```python
from build123d import *

# Parameters (mm, degrees)
PAD036_DEPTH            = 1.8
SKETCH112_R             = 2.25
PAD037_DEPTH            = 2.6
CHAMFER001_SIZE         = 0.4
SKETCH113_W             = 1.4
SKETCH113_H             = 2
SKETCH113_W_2           = 6.443533
SKETCH113_H_2           = 0.4
SKETCH113_W_3           = 7.136163
POCKET007_DEPTH         = 1.8
CHAMFER005_SIZE         = 0.2
BODY035_PLACEMENT_ANGLE = 23.8


with BuildPart() as part:
    # Sketch111 → Pad036 (new body)
    with BuildSketch(Plane.YZ):
        with BuildLine():
            Line((-6.5, 2.25), (-6.5, -2.25))
            ThreePointArc((-6.5, -2.25), (-6.207107, -2.957107), (-5.5, -3.25))
            Line((-5.5, -3.25), (5.5, -3.25))
            ThreePointArc((5.5, -3.25), (6.207107, -2.957107), (6.5, -2.25))
            Line((6.5, -2.25), (6.5, 2.25))
            ThreePointArc((6.5, 2.25), (6.207107, 2.957107), (5.5, 3.25))
            Line((-5.5, 3.25), (5.5, 3.25))
            ThreePointArc((-5.5, 3.25), (-6.207107, 2.957107), (-6.5, 2.25))
        make_face()
    extrude(amount=PAD036_DEPTH)

    # Sketch112 (on Face9 of Pad036) → Pad037 (join)
    with BuildSketch(Plane(origin=(0, 0, 0), x_dir=(0, 1, 0), z_dir=(-1, 0, 0))):
        Circle(SKETCH112_R)
    extrude(amount=PAD037_DEPTH)

    # Chamfer001
    chamfer001_edges = [part.edges().sort_by_distance(p)[0] for p in [
        (-2.6, -2.25, 0),
    ]]
    chamfer(chamfer001_edges, length=CHAMFER001_SIZE)

    # Sketch113 (on Face13 of Chamfer001) → Pocket007 (cut)
    with BuildSketch(Plane.YZ.offset(1.8)):
        with Locations((-0.008084, 2.25)):
            Rectangle(SKETCH113_W, SKETCH113_H)
        with Locations((4.913683, 3.05)):
            Rectangle(SKETCH113_W_2, SKETCH113_H_2)
        with Locations((-5.276165, 3.05)):
            Rectangle(SKETCH113_W_3, SKETCH113_H_2)
    extrude(amount=-POCKET007_DEPTH, mode=Mode.SUBTRACT)

    # Chamfer005
    chamfer005_edges = [part.edges().sort_by_distance(p)[0] for p in [
        (1.8, -0.708084, 2.25),
        (1.8, 0.691916, 2.25),
        (0.9, 0.691916, 3.25),
        (0.9, -0.708084, 3.25),
    ]]
    chamfer(chamfer005_edges, length=CHAMFER005_SIZE)


with BuildPart() as part_1:
    # Body035 placement: moved
    add(part.part.moved(Location((-19.5, 50, -6.9))).rotate(Axis((-19.5, 50, -6.9), (0, 0, -1)), BODY035_PLACEMENT_ANGLE))


solid = part_1.part
```
Design review of the part built by this model. Coordinates are the model's own, in mm. A direction names the side the tool comes from. Give positions to 0.01 mm unless a question says otherwise; leave off trailing zeros. Loops run counter-clockwise (first coordinate to the right, second up) from the corner with the lowest first, then second, coordinate; pieces in that order, holes last. Notation, with made-up numbers: (60, -30.5) -> (94, -30.5) arc R12 cw to (94, -24.5) -> close; hole circle Ø4 at (87, 84.5). An arc over 180 degrees is marked (long way). One line per item, written item: value.
Q1. We need section C-C on z = -9.5. Give the boundary of the cut face in (x, y).
Numbers:
outline: (-22.1, 44.11) -> (-20.45, 43.38) -> (-15.26, 55.16) -> (-16.9, 55.89) -> close
Q2. Machinability: for faces 4 (the flat face through (-18.479, 50.306, -4.763)), 5 (the flat face through (-21.311, 43.695, -6.869)), which of the approach directions +Z, -Z, +X, -X, +Y, -Y give a long, thin tool a straight path to every point of the face, cutting with its end or side? Answer none if there is none.
Numbers:
face 4: +Z
face 5: +Z, -Z, -X, -Y
Q3. For L1, parallel to Z at x = -20.5, y = 45.5; L2, parallel to Y at x = -18.5, z = -4; L3, parallel to Y at x = -21.5, z = -4.25, list the stretches that pass through material, from the lowest coordinate up.
Numbers:
L1: z = -10.15 to -4.05
L2: y = 47.81 to 48.79, 50.32 to 51.41
L3: y = 43.87 to 45.47
Q4. Draft analysis for pull direction X (two halves, no side actions). For faces 1 (the flat face through (-16.07, 55.59, -6.93)), 2 (the flat face through (-19, 50, -10.15)), 3 (the flat face through (-19, 50, -5.65)), state which applies: pulls with the +X half, pulls with the -X half, needs draft (parallel to the pull), parting line crosses it, or undercut.
Numbers:
face 1: pulls with the +X half
face 2: needs draft
face 3: undercut
Q5. We need section A-A on z = -4.25. Give the boundary of the cut face in (x, y).
Numbers:
outline: (-22.09, 44.13) -> (-20.44, 43.4) -> (-18.22, 48.44) -> (-18.32, 48.71) -> (-19.79, 49.35) -> close; (-19.22, 50.63) -> (-17.76, 49.99) -> (-17.49, 50.09) -> (-15.26, 55.14) -> (-16.91, 55.87) -> close
Q6. For pin 1 Ø2 at (y, z) = (45, -6) entering from +X; pin 2 Ø1.5 at (x, z) = (-18, -7.5) entering from +Y; pin 3 Ø1.7 at (x, y) = (-20.5, 46.5) entering from +Z; pin 4 Ø1.1 at (x, y) = (-18.5, 49) entering from +Z, all flat-tipped, find the tip position at first contact; note any pin that passes through.
Numbers:
pin 1: stops at x = -19.3
pin 2: stops at y = 55.1
pin 3: stops at z = -4.05
pin 4: stops at z = -3.65
Q7. We need section B-B on y = 47.5. Give the boundary of the cut face in (x, z), and give its area (3 significant figures).
Numbers:
outline: (-20.6, -10.15) -> (-18.64, -10.15) -> (-18.64, -4.05) -> (-20.6, -4.05) -> close
area: 12.0 mm^2
